For this review, take the finished solid that the model builds, in its own axes (mm). A direction names the side the tool comes from. Round coordinates to 2 decimals unless told otherwise and drop trailing zeros. Write each loop counter-clockwise with the first axis right and the second up, starting at its lowest first coordinate (ties: lowest second). Pieces come first, ordered by that corner, then holes.
from build123d import *

# Parameters (mm, degrees)
BOSS_EXTRUDE1_DEPTH = 44.25
BOSS_EXTRUDE2_DEPTH = 39
BOSS_EXTRUDE3_DEPTH = 39
LPATTERN1_START     = 0.1
LPATTERN1_DEPTH     = 39
SPLIT1_START        = 0.1
SPLIT1_DEPTH        = 39
SPLIT1_2_DEPTH      = 39
SPLIT1_3_DEPTH      = 39


# Read off the part's stored shape, not the designer's step: LPattern1, Split1
with BuildPart() as part:
    # Sketch1 → Boss-Extrude1 (new body)
    with BuildSketch(Plane.XY):
        Polygon((-14.81, 0.1), (-15.885, 0.1), (-15.885, -2.1), (-13.345, -2.1), (-13.345, -3.06), (-16.845, -3.06), (-16.845, 1.06), (-15.77, 1.06), (-15.77, 40.06), (0, 40.06), (15.77, 40.06), (15.77, 1.06), (16.845, 1.06), (16.845, -3.06), (13.345, -3.06), (13.345, -2.1), (15.885, -2.1), (15.885, 0.1), (14.81, 0.1), (14.81, 39.1), (0, 39.1), (-14.81, 39.1), align=None)
    extrude(amount=-BOSS_EXTRUDE1_DEPTH)

    # Sketch2 → Boss-Extrude2 (add)
    with BuildSketch(Plane.XZ.offset(-39.1)):
        Polygon((-14.81, -2.66), (-13.81, -2.66), (-14.81, -3.66), align=None)
        Polygon((14.81, -3.66), (14.81, -2.66), (13.81, -2.66), align=None)
    extrude(amount=BOSS_EXTRUDE2_DEPTH)

    # Sketch3 → Boss-Extrude3 (add)
    with BuildSketch(Plane.XZ.offset(-39.1)):
        Polygon((-14.81, -32.99), (-14.81, -38.01), (-13.65, -36.85), (-14.15, -36.35), (-14.15, -34.65), (-13.65, -34.15), align=None)
        Polygon((14.15, -36.35), (13.65, -36.85), (14.81, -38.01), (14.81, -32.99), (13.65, -34.15), (14.15, -34.65), align=None)
    extrude(amount=BOSS_EXTRUDE3_DEPTH)

    # LPattern1 outline → LPattern1 (add)
    with BuildSketch(Plane(origin=(0, 0, 0), x_dir=(1, 0, 0), z_dir=(0, 1, 0)).offset(LPATTERN1_START)):
        Polygon((-13.65, 20.85), (-14.81, 22.01), (-14.81, 16.99), (-13.65, 18.15), (-14.15, 18.65), (-14.15, 20.35), align=None)
        Polygon((-14.15, 26.65), (-14.15, 28.35), (-13.65, 28.85), (-14.81, 30.01), (-14.81, 24.99), (-13.65, 26.15), align=None)
        Polygon((-14.15, 41.65), (-14.15, 43.35), (-13.65, 43.85), (-14.81, 45.01), (-14.81, 39.99), (-13.65, 41.15), align=None)
        Polygon((14.81, 16.99), (14.81, 22.01), (13.65, 20.85), (14.15, 20.35), (14.15, 18.65), (13.65, 18.15), align=None)
        Polygon((14.15, 28.35), (14.15, 26.65), (13.65, 26.15), (14.81, 24.99), (14.81, 30.01), (13.65, 28.85), align=None)
        Polygon((14.15, 43.35), (14.15, 41.65), (13.65, 41.15), (14.81, 39.99), (14.81, 45.01), (13.65, 43.85), align=None)
    extrude(amount=LPATTERN1_DEPTH)

    # Split1 outline → Split1 (cut)
    with BuildSketch(Plane(origin=(0, 0, 0), x_dir=(1, 0, 0), z_dir=(0, 1, 0)).offset(SPLIT1_START)):
        Polygon((14.81, 45.01), (14.05, 44.25), (14.81, 44.25), align=None)
        Polygon((-14.05, 44.25), (-14.81, 45.01), (-14.81, 44.25), align=None)
    extrude(amount=SPLIT1_DEPTH, mode=Mode.SUBTRACT)


with BuildPart() as body_2:
    # Split1 2 outline → Split1 2 (new body)
    with BuildSketch(Plane(origin=(0, 0, 0), x_dir=(1, 0, 0), z_dir=(0, 1, 0)).offset(SPLIT1_START)):
        Polygon((-14.81, 44.25), (-14.05, 44.25), (-14.81, 45.01), align=None)
    extrude(amount=SPLIT1_2_DEPTH)


with BuildPart() as body_3:
    # Split1 3 outline → Split1 3 (new body)
    with BuildSketch(Plane(origin=(0, 0, 0), x_dir=(1, 0, 0), z_dir=(0, 1, 0)).offset(SPLIT1_START)):
        Polygon((14.05, 44.25), (14.81, 44.25), (14.81, 45.01), align=None)
    extrude(amount=SPLIT1_3_DEPTH)


solid = part.part
(1) For faces 1 (the face through (14.2, 19.3, -17.6)), 2 (the face through (-15, -3.06, -22)), 3 (the face through (-14.81, 20, -1)), list the 3-axis set-ups (+Z, -Z, +X, -X, +Y, -Y) from which the entire face can be reached by the end or side of a thin tool; tool diameter is ignored.
Geometry check:
face 1: none
face 2: +Z, -Z, +X, -X, -Y
face 3: +Z
(2) For pin 1 Ø3 at (y, z) = (14, -39.5) entering from -X; pin 2 Ø1.5 at (y, z) = (17, -6.5) entering from +X; pin 3 Ø12 at (x, z) = (-12.5, -27) entering from -Y; pin 4 Ø1.1 at (x, y) = (-14, 16.5) entering from +Z, all flat-tipped, find the tip position at first contact; note any pin that passes through.
Geometry check:
pin 1: stops at x = -15.77
pin 2: stops at x = 15.77
pin 3: stops at y = -3.06
pin 4: stops at z = -2.66
(3) We need section B-B, the plane x = 8. Give the boundary of the cut face in (y, z).
Geometry check:
outline: (39.1, -44.25) - (40.06, -44.25) - (40.06, 0) - (39.1, 0) - close
(4) For line 1 along X through (y, z) = (0.5, -8) (3 decimals); line 2 along X through (y, z) = (27.5, -37); line 3 along Y through (x, z) = (-14.5, -39), list the stretches that pass through material, from the lowest coordinate up.
Geometry check:
line 1: x = -16.845 to -14.81, 14.81 to 16.845
line 2: x = -15.77 to -13.8, 13.8 to 15.77
line 3: y = -3.06 to -2.1, 39.1 to 40.06
(5) We need section A-A, the plane z = -16. Give the boundary of the cut face in (x, y) (3 decimals), and give its area (3 significant figures).
Geometry check:
outline: (-16.845, -3.06) - (-13.345, -3.06) - (-13.345, -2.1) - (-15.885, -2.1) - (-15.885, 0.1) - (-14.81, 0.1) - (-14.81, 39.1) - (14.81, 39.1) - (14.81, 0.1) - (15.885, 0.1) - (15.885, -2.1) - (13.345, -2.1) - (13.345, -3.06) - (16.845, -3.06) - (16.845, 1.06) - (15.77, 1.06) - (15.77, 40.06) - (-15.77, 40.06) - (-15.77, 1.06) - (-16.845, 1.06) - close
area: 118 mm2
(6) Mouldability with a two-part tool opening along Z and no side actions: class faces 4 (the face through (15, -3.06, -22)), 5 (the face through (-14.2, 19.3, -17.6)) as pulls with the +Z half, pulls with the -Z half, needs draft (parallel to the pull), parting line crosses it, or undercut.
Geometry check:
face 4: needs draft
face 5: undercut
